Design review of the part built by this model. Coordinates are the model's own, in mm. Face numbers are marked on the shaded views. A direction names the side the tool comes from. Coordinates: 2 decimals unless noted, no trailing zeros. Write each loop counter-clockwise with the first axis right and the second up, starting at its lowest first coordinate (ties: lowest second). Pieces come first, ordered by that corner, then holes.
```python
from build123d import *

# Parameters (mm, degrees)
SKETCH1_W                 = 21
SKETCH1_H                 = 45
BOSS_EXTRUDE1_DEPTH       = 40
CHAMFER1_SIZE             = 60
CHAMFER1_SIZE_2           = 16.076951546
SKETCH2_W                 = 3
SKETCH2_H                 = 45
CUT_EXTRUDE1_DEPTH        = 1.6
F_6_32_TAPPED_HOLE1_D     = 2.7051
F_6_32_TAPPED_HOLE1_DEPTH = 9
F_6_32_TAPPED_HOLE1_TIP   = 0.81269403
CHAMFER2_SIZE             = 5
CHAMFER2_SIZE2            = 18.660254038
SKETCH11_R                = 1.63195
CUT_EXTRUDE3_DEPTH        = 10
F_3DSKETCH1_R             = 2.794
CUT_EXTRUDE4_DEPTH        = 8
SKETCH12_W                = 6
SKETCH12_H                = 45
CUT_EXTRUDE5_DEPTH        = 0.5


with BuildPart() as part:
    # Sketch1 → Boss-Extrude1 (new body)
    with BuildSketch(Plane(origin=(0, 0, 0), x_dir=(1, 0, 0), z_dir=(0, 1, 0))):
        Rectangle(SKETCH1_W, SKETCH1_H)
    extrude(amount=-BOSS_EXTRUDE1_DEPTH)

    # Chamfer1
    # the kernel refuses this chamfer: 60, 16.076951546 mm, written as the material it takes off along each edge
    with BuildSketch(Plane(origin=(10.5, 0, 178.303294212), x_dir=(0.009967146577156426, -0.9999503267608394, 0), z_dir=(0, 0, -1))) as chamfer1_piece_1:
        Polygon((CHAMFER1_SIZE * 0.999950326761, CHAMFER1_SIZE * 0.00996714657716), (-CHAMFER1_SIZE_2 * 0.00996714657707, CHAMFER1_SIZE_2 * 0.999950326753), (0, 0), align=None)
    extrude(amount=356.606588424, mode=Mode.SUBTRACT)

    # Sketch2 → Cut-Extrude1 (cut)
    with BuildSketch(Plane(origin=(-5.20336663, -1.394237886, 0), x_dir=(0, 0, -1), z_dir=(0.965925826289069, 0.2588190451025185, 0))):
        with Locations((0, -19.262102335)):
            Rectangle(SKETCH2_W, SKETCH2_H)
    extrude(amount=-CUT_EXTRUDE1_DEPTH, mode=Mode.SUBTRACT)

    # #6-32 Tapped Hole1
    with Locations(Plane(origin=(-5.20336663, -1.394237886, 0), x_dir=(0, 0, -1), z_dir=(0.965925826289069, 0.2588190451025185, 0))):
        with Locations((-20, -20.93024544), (20, -20.93024544), (-20, -5.93024544), (-20, -35.93024544), (20, -35.93024544), (20, -5.93024544)):
            Hole(F_6_32_TAPPED_HOLE1_D / 2, depth=F_6_32_TAPPED_HOLE1_DEPTH)
            with Locations((0, 0, -(F_6_32_TAPPED_HOLE1_DEPTH + F_6_32_TAPPED_HOLE1_TIP / 2))):  # 118° drill point
                Cone(0, F_6_32_TAPPED_HOLE1_D / 2, F_6_32_TAPPED_HOLE1_TIP, mode=Mode.SUBTRACT)

    # Chamfer2
    chamfer2_edges = [part.edges().sort_by_distance(p)[0] for p in [
        (-10.5, -40, 0),
    ]]
    chamfer2_side = [part.faces().sort_by_distance(p)[0] for p in [
        (-2.729210232, -40, 0),
    ]]
    chamfer(chamfer2_edges, length=CHAMFER2_SIZE, length2=CHAMFER2_SIZE2, reference=chamfer2_side[0])

    # Sketch11 → Cut-Extrude3 (cut)
    with BuildSketch(Plane(origin=(-10.5, 29.282032303, 0), x_dir=(0, 0, 1), z_dir=(1, 0, 0))):
        with Locations(Location((8.89, 33.551905284, 0), (0, 0, 270))):
            Circle(SKETCH11_R)
        with Locations((8.89, 46.351905284)):
            Circle(SKETCH11_R)
        with Locations(Location((-8.89, 46.351905284, 0), (0, 0, 270))):
            Circle(SKETCH11_R)
        with Locations((-8.89, 33.551905284)):
            Circle(SKETCH11_R)
    extrude(amount=CUT_EXTRUDE3_DEPTH, mode=Mode.SUBTRACT)

    # 3DSketch1 → Cut-Extrude4 (cut)
    with BuildSketch(Plane(origin=(-7.5, -4.269872981, -8.91), x_dir=(0, -0.5834969796278836, 0.812115308786343), z_dir=(-1, 0, 0))):
        with Locations(Location((0, 0, 0), (0, 0, 305.696879334))):
            Circle(F_3DSKETCH1_R)
        with Locations(Location((14.471894803, 10.397916177, 0), (0, 0, 305.696879334))):
            Circle(F_3DSKETCH1_R)
        with Locations(Location((21.942696816, 0, 0), (0, 0, 305.696879334))):
            Circle(F_3DSKETCH1_R)
        with Locations(Location((7.470802013, -10.397916177, 0), (0, 0, 305.696879334))):
            Circle(F_3DSKETCH1_R)
    extrude(amount=-CUT_EXTRUDE4_DEPTH, mode=Mode.SUBTRACT)

    # Sketch12 → Cut-Extrude5 (cut)
    with BuildSketch(Plane(origin=(-5.20336663, -1.394237886, 0), x_dir=(0, 0, -1), z_dir=(0.9659258262890663, 0.25881904510252807, 0))):
        with Locations((0, -20.203205195)):
            Rectangle(SKETCH12_W, SKETCH12_H)
    extrude(amount=-CUT_EXTRUDE5_DEPTH, mode=Mode.SUBTRACT)


solid = part.part
```
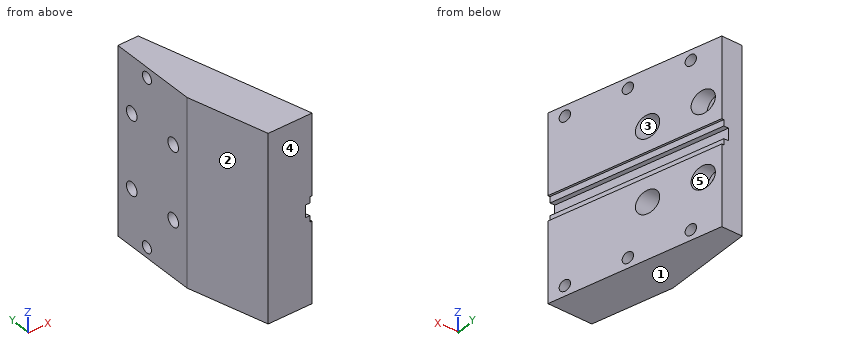
(1) Mouldability with a two-part tool opening along Z and no side actions: class the marked faces 1, 2 and 3 as +Z half, -Z half, draft (parallel to the pull), parting line (faces both ways), or undercut.
(2) Wall thickness on line 1 (Z direction, x = 1.5, y = -31); line 2 (Z direction, x = 2, y = -35.5); line 3 (X direction, y = -27, z = -20): over which ranges is each line inside the solid? List them lowest first.
(3) Consider section D-D (x = -1). State how many separate pieces and enclosed holes the cut face has, plus the area to 3 significant figures.
(4) For the marked faces 4 and 5, list the 3-axis set-ups (+Z, -Z, +X, -X, +Y, -Y) from which the entire face can be reached by the end or side of a thin tool; tool diameter is ignored.
(5) Consider section B-B (z = -13). Give the boundary of the cut face in (x, y), plus the area to 3 significant figures.
(6) Consider section A-A (z = -8). Give the boundary of the cut face in (x, y), plus the area to 3 significant figures.
(7) Insertion check: pin 1 Ø4.5 at (y, z) = (-4, -9) entering from +X; pin 2 Ø2 at (y, z) = (-31, -12) entering from +X; pin 3 Ø6.5 at (y, z) = (-17.07, -8.91) entering from +X; pin 4 Ø1.7 at (y, z) = (-17.5, -9.5) entering from +X. Each pin has a flat end and moves straight along its axis. Give the tip position at first contact, or say it passes through.
(8) Consider section C-C (y = -11). Give the boundary of the cut face in (x, z), plus the area to 3 significant figures.
Results:
1. face 1: -Z half
1. face 2: draft
1. face 3: undercut
2. line 1: z = -22.5 to -1.5, 1.5 to 22.5
2. line 2: z = -22.5 to -20.75, -19.25 to 19.25, 20.75 to 22.5
2. line 3: x = -8.98 to 1.66
3. separate pieces: 1
3. enclosed holes: 4
3. area: 959 mm2
4. face 4: +Z, -Z, +X, -X, -Y
4. face 5: +X
5. outline: (-10.5, -21.34) - (-5.5, -40) - (5.14, -40) - (-5.58, 0) - (-10.5, 0) - close
5. area: 365 mm2
6. outline: (-10.5, -21.34) - (-5.5, -40) - (5.14, -40) - (-0.29, -19.72) - (-7.5, -19.72) - (-7.5, -18.44) - (-10.5, -18.44) - close; (-10.5, -15.7) - (-7.5, -15.7) - (-7.5, -14.43) - (-1.71, -14.43) - (-3.73, -6.91) - (-7.5, -6.91) - (-7.5, -5.64) - (-10.5, -5.64) - close; (-10.5, -2.9) - (-7.5, -2.9) - (-7.5, -1.63) - (-5.14, -1.63) - (-5.58, 0) - (-10.5, 0) - close
6. area: 298 mm2
7. pin 1: stops at x = -7.5
7. pin 2: stops at x = 3
7. pin 3: stops at x = -0.13
7. pin 4: passes through
8. outline: (-10.5, -22.5) - (-2.63, -22.5) - (-2.63, -3) - (-3.15, -3) - (-3.15, -1.5) - (-4.29, -1.5) - (-4.29, 1.5) - (-3.15, 1.5) - (-3.15, 3) - (-2.63, 3) - (-2.63, 22.5) - (-10.5, 22.5) - close
8. area: 348 mm2
